Input: part model. Units: mm. Frame: model coordinates. Round coordinates to 2 decimals unless told otherwise and drop trailing zeros. Write each loop counter-clockwise with the first axis right and the second up, starting at its lowest first coordinate (ties: lowest second). Pieces come first, ordered by that corner, then holes. Notation, with made-up numbers: (43, 6) -> (52, 6) arc R37 cw to (52, 45) -> close; hole circle Ø9 at (42, -8.5). An arc over 180 degrees is marked (long way). Write item = value, one per line.
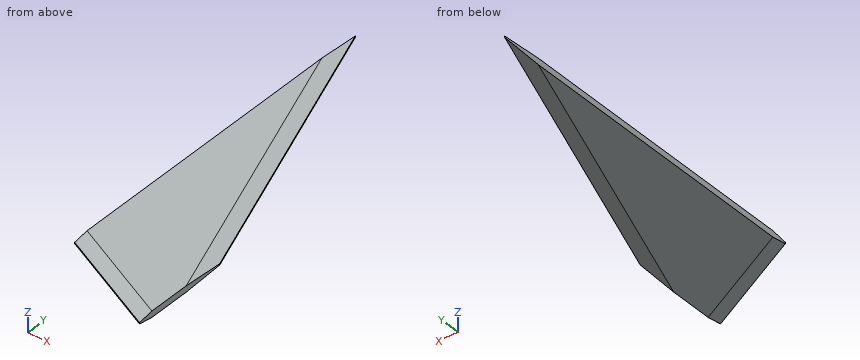
```python
from build123d import *
from OCP.BRepFilletAPI import BRepFilletAPI_MakeChamfer

# Parameters (mm, degrees)
BOSS_EXTRUDE1_DEPTH = 1.5875
CHAMFER1_SIZE       = 1.25
CHAMFER1_SIZE2      = 7.089102275


with BuildPart() as part:
    # Sketch1 → Boss-Extrude1 (new, symmetric)
    with BuildSketch(Plane.XY):
        Polygon((-16.410036231, -60.699177334), (-16.410036231, 117.100822666), (37.564963769, -35.299177334), (37.564963769, -86.099177334), align=None)
    extrude(amount=BOSS_EXTRUDE1_DEPTH, both=True)

    # Chamfer1: one chamfer whose edges measure the first distance from different faces: ONE call of the kernel's chamfer builder (chamfer() names one face for all edges)
    chamfer1_edges_1 = [part.edges().sort_by_distance(p)[0] for p in [
        (10.577463769, 40.900822666, 1.5875),
        (10.577463769, 40.900822666, -1.5875),
    ]]
    chamfer1_side_1 = [part.faces().sort_by_distance(p)[0] for p in [
        (10.577463769, 40.900822666, 0),
    ]]
    chamfer1_edges_2 = [part.edges().sort_by_distance(p)[0] for p in [
        (10.577463769, -73.399177334, 1.5875),
        (10.577463769, -73.399177334, -1.5875),
    ]]
    chamfer1_side_2 = [part.faces().sort_by_distance(p)[0] for p in [
        (10.577463769, -73.399177334, 0),
    ]]
    chamfer1 = BRepFilletAPI_MakeChamfer(part.part.solid().wrapped)
    for e in chamfer1_edges_1:
        chamfer1.Add(CHAMFER1_SIZE, CHAMFER1_SIZE2, e.wrapped, chamfer1_side_1[0].wrapped)  # the first distance lies on this face
    for e in chamfer1_edges_2:
        chamfer1.Add(CHAMFER1_SIZE, CHAMFER1_SIZE2, e.wrapped, chamfer1_side_2[0].wrapped)  # the first distance lies on this face
    add(Compound.cast(chamfer1.Shape()), mode=Mode.REPLACE)


solid = part.part
```
1) Cut plane D-D (x = 5). Return the cut outline in (y, z), and give its area (3 significant figures).
Solutions:
outline = (-70.77, -0.34) -> (-62.94, -1.59) -> (35.41, -1.59) -> (56.65, -0.34) -> (56.65, 0.34) -> (35.41, 1.59) -> (-62.94, 1.59) -> (-70.77, 0.34) -> close
area = 368 mm^2
2) Cut plane A-A (x = -4). Return the cut outline in (y, z), and give its area (3 significant figures).
Solutions:
outline = (-66.54, -0.34) -> (-58.7, -1.59) -> (60.83, -1.59) -> (82.06, -0.34) -> (82.06, 0.34) -> (60.83, 1.59) -> (-58.7, 1.59) -> (-66.54, 0.34) -> close
area = 435 mm^2
3) Cut plane B-B (y = -17.5). Return the cut outline in (x, z).
Solutions:
outline = (-16.41, -1.59) -> (23.74, -1.59) -> (31.26, -0.34) -> (31.26, 0.34) -> (23.74, 1.59) -> (-16.41, 1.59) -> close
4) Cut plane C-C (z = 1.1). Return the cut outline in (x, y), and give its area (3 significant figures).
Solutions:
outline = (-16.41, -55.92) -> (37.56, -81.32) -> (37.56, -48.25) -> (-16.41, 104.15) -> close
area = 5,210 mm^2
5) Line query: L1, parallel to X at y = 46, z = 0.25; L2, parallel to Z at x = -8, y = 73; L3, parallel to X at y = 54, z = 0.3. Output: solid intervals per line, ascending. Write a range as from..to.
Solutions:
L1 = -16.41..8.77
L2 = -1.54..1.54
L3 = -16.41..5.94
6) First-contact query: P1, Ø1, axis at y = -2.5, z = 0.5, coming from the +X side. Flat tip, straight axial feed; report the tip coordinate or a pass-through.
Solutions:
P1 = 26.12
